The listing builds one solid part. Answer for the finished solid, in the listing's coordinates (mm). Face numbers are marked on the shaded views. A direction names the side the tool comes from. Round coordinates to 2 decimals unless told otherwise and drop trailing zeros. Loops run counter-clockwise (first coordinate to the right, second up) from the corner with the lowest first, then second, coordinate; pieces in that order, holes last. Notation, with made-up numbers: M 79,-37 L 95,-37 A11 cw 95,-26 Z; hole C -17,54 d6. An arc over 180 degrees is marked long. Answer as a JSON object with one key per item and string values.
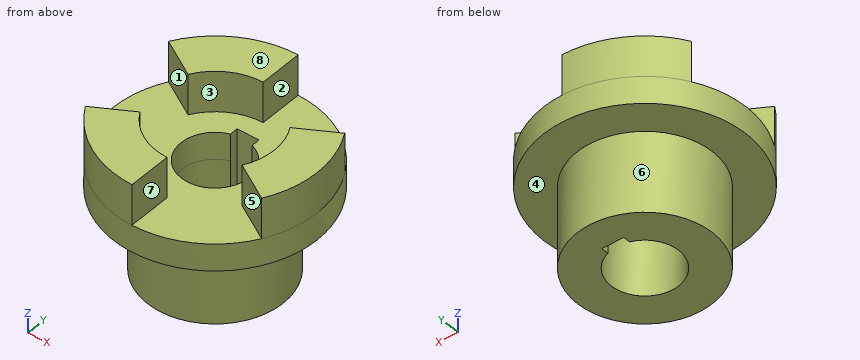
```python
from build123d import *
from build123d.topology import SkipClean

# Parameters (mm, degrees)
SKETCH1_R           = 37.5
BOSS_EXTRUDE1_DEPTH = 10
BOSS_EXTRUDE2_DEPTH = 15
BOSS_EXTRUDE3_START = 30
SKETCH5_R           = 25
SKETCH5_R_2         = 12.5
BOSS_EXTRUDE3_DEPTH = 30
CUT_EXTRUDE1_DEPTH  = 4


with BuildPart() as part:
    # Sketch1 → Boss-Extrude1 (new body)
    with BuildSketch(Plane.XY):
        Circle(SKETCH1_R)
        with BuildLine():
            ThreePointArc((-4, 11.842719282), (0, -12.5), (4, 11.842719282))
            ThreePointArc((4, 11.842719282), (0, 12.5), (-4, 11.842719282))
        make_face(mode=Mode.SUBTRACT)
    extrude(amount=BOSS_EXTRUDE1_DEPTH)

    # Sketch3 → Boss-Extrude2 (add)
    with SkipClean():  # the faces are left unmerged after this step: merging them gives an invalid solid
        with BuildSketch(Plane.XY.offset(10)):
            with BuildLine():
                Line((-32.475952642, -18.75), (-18.798362826, -10.853239838))
                ThreePointArc((-18.798362826, -10.853239838), (-10.853239838, -18.798362826), (0, -21.706479676))
                Line((0, -21.706479676), (0, -37.5))
                ThreePointArc((0, -37.5), (-18.75, -32.475952642), (-32.475952642, -18.75))
            make_face()
            with BuildLine():
                Line((0, 37.5), (0, 21.706479676))
                ThreePointArc((0, 21.706479676), (-10.853239838, 18.798362826), (-18.798362826, 10.853239838))
                Line((-18.798362826, 10.853239838), (-32.475952642, 18.75))
                ThreePointArc((-32.475952642, 18.75), (-18.75, 32.475952642), (0, 37.5))
            make_face()
            with BuildLine():
                Line((32.475952642, -18.75), (18.798362826, -10.853239838))
                ThreePointArc((18.798362826, -10.853239838), (21.706479676, 0), (18.798362826, 10.853239838))
                Line((18.798362826, 10.853239838), (32.475952642, 18.75))
                ThreePointArc((32.475952642, 18.75), (37.5, 0), (32.475952642, -18.75))
            make_face()
        extrude(amount=BOSS_EXTRUDE2_DEPTH)

    # Sketch5 → Boss-Extrude3 (add)
    with SkipClean():  # the faces are left unmerged after this step: merging them gives an invalid solid
        with BuildSketch(Plane(origin=(0, 0, 0), x_dir=(-1, 0, 0), z_dir=(0, 0, -1)).offset(BOSS_EXTRUDE3_START)):
            with Locations(Location((0, 0, 0), (0, 0, 180))):
                Circle(SKETCH5_R)
            Circle(SKETCH5_R_2, mode=Mode.SUBTRACT)
        extrude(amount=-BOSS_EXTRUDE3_DEPTH)

    # Sketch7 → Cut-Extrude1 (cut, symmetric)
    with SkipClean():  # the faces are left unmerged after this step: merging them gives an invalid solid
        with BuildSketch(Plane(origin=(0, 0, 0), x_dir=(0, 0, -1), z_dir=(1, 0, 0))):
            Polygon((30, 0), (-10, 0), (-10, 14.9), (30, 14.5), align=None)
        extrude(amount=CUT_EXTRUDE1_DEPTH, both=True, mode=Mode.SUBTRACT)


solid = part.part
```
Item 1: Straight lines are drawn through the part: line 1 (X direction, y = 0, z = 4.5); line 2 (Y direction, x = 11, z = -24); line 3 (Z direction, x = -28, y = 3). For each, find the intervals that lie inside material, in ascending order.
Values follow:
{"line 1": "-37.5 to -12.5, 12.5 to 37.5", "line 2": "-22.45 to -5.94, 5.94 to 22.45", "line 3": "0 to 10"}
Item 2: The part is cut by section B-B (z = 18). Give the vertices of the cut face in (x, y), then the cut area to 3 significant figures.
Values follow:
{"outline": "M -32.48,-18.75 A37.5 ccw 0,-37.5 L 0,-21.71 A21.71 cw -18.8,-10.85 Z; M -32.48,18.75 L -18.8,10.85 A21.71 cw 0,21.71 L 0,37.5 A37.5 ccw Z; M 18.8,-10.85 L 32.48,-18.75 A37.5 ccw 32.48,18.75 L 18.8,10.85 A21.71 cw Z", "area": "1,470 mm^2"}
Item 3: Determine the mould class of the marked faces 5, 6, 7 and 8 for opening direction X: released by +X, released by -X, zero draft, split by the parting line, or undercut.
Values follow:
{"face 5": "undercut", "face 6": "split by the parting line", "face 7": "released by +X", "face 8": "zero draft"}
Item 4: Which of the six approach directions +Z, -Z, +X, -X, +Y, -Y give full straight-line access (tool end or side, diameter ignored) to the marked faces 1, 2, 3 and 4?
Values follow:
{"face 1": "+Z, -X", "face 2": "+Z, +X, +Y, -Y", "face 3": "+Z", "face 4": "-Z"}
Item 5: The part is cut by section D-D (z = -11). Give the vertices of the cut face in (x, y).
Values follow:
{"outline": "C 0,0 d50; hole M -4,11.84 A12.5 ccw long 4,11.84 L 4,14.69 L -4,14.69 Z"}
Item 6: The part is cut by section A-A (y = 0). Give the vertices of the cut face in (x, z), then the cut area to 3 significant figures.
Values follow:
{"outline": "M -37.5,0 L -25,0 L -25,-30 L -12.5,-30 L -12.5,10 L -37.5,10 Z; M 12.5,-30 L 25,-30 L 25,0 L 37.5,0 L 37.5,25 L 21.71,25 L 21.71,10 L 12.5,10 Z", "area": "1,490 mm^2"}
Item 7: Flat-ended cylindrical pins translate along their axes: P1, Ø3, axis at x = 16, y = -25, coming from the +Z side; P2, Ø6, axis at x = -28.5, z = -17, coming from the -Y side; P3, Ø12, axis at y = -29, z = 18.5, coming from the +X side; P4, Ø2.5, axis at y = 13, z = -11.5, coming from the -X side. Find the tip coordinate at first contact, or state that the pin passes through.
Values follow:
{"P1": "z = 10", "P2": "through", "P3": "x = 0", "P4": "x = -22.07"}
Item 8: The part is cut by section C-C (x = -3). Give the vertices of the cut face in (y, z).
Values follow:
{"outline": "M -37.38,0 L -24.82,0 L -24.82,-30 L -12.13,-30 L -12.13,10 L -21.5,10 L -21.5,25 L -37.38,25 Z; M 14.5,-30 L 24.82,-30 L 24.82,0 L 37.38,0 L 37.38,25 L 21.5,25 L 21.5,10 L 14.9,10 Z"}
